Model file for the job. Use its own axes, mm. A direction names the side the tool comes from. Give positions to 0.01 mm unless a question says otherwise; leave off trailing zeros. Order: outer loops, then holes, each group sorted by start corner. A loop starts at its lowest first (then second) coordinate and runs counter-clockwise, first axis right, second up. Notation, with made-up numbers: M 26,7.25 L 76,7.25 A29 cw 76,35.25 Z; hole C 60.25,40 d10. An arc over 180 degrees is marked long. Return JSON: item names as keys, results as strings. Group by question number.
1. Slice it at B-B on z = 3.75. List the corners of the cut face in (x, y), then the cut area to 3 significant figures.
2. Two-plate mould, pull along Y, no slides. Class faces 1 (the face through (0, 42.5, 12)), 2 (the face through (26, -1, 10)), 3 (the face through (0, -1, 18)): released by +Y, released by -Y, zero draft, split by the parting line, or undercut.
3. 3-axis set-ups, long thin cutter, end or side, ignore diameter. For faces 4 (the face through (25, 1, -1)), 5 (the face through (0, 1, 20)), 6 (the face through (-25, 1, -1)), 7 (the face through (-6, -41.5, 15)): which of +Z, -Z, +X, -X, +Y, -Y reach the whole face in a straight line?
4. Pin check, flat tips, straight feed: pin 1 (0.5 mm diameter, centred on x = -3.5, y = 42, fed in from -Z); pin 2 (1.1 mm diameter, centred on x = -24.5, z = -1.5, fed in from -Y); pin 3 (4 mm diameter, centred on x = 3.5, z = 12.5, fed in from -Y). Stop position of each tip, or through.
5. Slice it at C-C on y = -8.5. List the corners of the cut face in (x, z).
6. Slice it at A-A on x = 17. List the corners of the cut face in (y, z), then the cut area to 3 significant figures.
7. Slice it at D-D on z = 11.5. List the corners of the cut face in (x, y).
8. Wall check: probe 1 along Y at (x, z) = (19, 17.75); probe 2 along X at (y, z) = (-7, 16); probe 3 along X at (y, z) = (20, -0.5). Give the ranges that are in metal, low to high. Write a range as [from, to].
from build123d import *

# Parameters (mm, degrees)
F0_W     = 52
F0_H     = 85
F1_DEPTH = 20
F2_W     = 48
F2_H     = 83
F3_DEPTH = 18
F4_W     = 1
F4_H     = 83
F5_DEPTH = 3
F7_DEPTH = 25
F9_DEPTH = 25


with BuildPart() as f1:
    # F0 (on Top) → F1 (new body)
    with BuildSketch(Plane.XY):
        Rectangle(F0_W, F0_H)
    extrude(amount=F1_DEPTH)

    # F2 (on face) → F3 (cut)
    with BuildSketch(Plane(origin=(0, 0, 0), x_dir=(1, 0, 0), z_dir=(0, 0, -1))):
        Rectangle(F2_W, F2_H)
    extrude(amount=-F3_DEPTH, mode=Mode.SUBTRACT)

    # F4 (on face) → F5 (join)
    with BuildSketch(Plane(origin=(0, 0, 0), x_dir=(1, 0, 0), z_dir=(0, 0, -1))):
        with Locations((-24.5, 0)):
            Rectangle(F4_W, F4_H)
        with Locations((24.5, 0)):
            Rectangle(F4_W, F4_H)
    extrude(amount=F5_DEPTH)

    # F6 (on face) → F7 (cut)
    with BuildSketch(Plane(origin=(0, 42.5, 0), x_dir=(-1, 0, 0), z_dir=(0, 1, 0))):
        Polygon((-20, 0), (0, 0), (20, 0), (20, 9), (-20, 9), align=None)
    extrude(amount=-F7_DEPTH, mode=Mode.SUBTRACT)

    # F8 (on face) → F9 (cut)
    with BuildSketch(Plane.XZ.offset(42.5)):
        with BuildLine():
            ThreePointArc((10.5, 5), (7.424621, 12.424621), (0, 15.5))
            ThreePointArc((0, 15.5), (-9.020809, 10.373546), (-9.233093, 0))
            Line((-9.233093, 0), (9.233093, 0))
            ThreePointArc((9.233093, 0), (10.178346, 2.420996), (10.5, 5))
        make_face()
    extrude(amount=-F9_DEPTH, mode=Mode.SUBTRACT)


solid = f1.part
Result:
{
 "1": {"outline": "M -26,-42.5 L -10.43,-42.5 L -10.43,-41.5 L -24,-41.5 L -24,41.5 L -20,41.5 L -20,42.5 L -26,42.5 Z; M 10.43,-42.5 L 26,-42.5 L 26,42.5 L 20,42.5 L 20,41.5 L 24,41.5 L 24,-41.5 L 10.43,-41.5 Z", "area": "375 mm2"},
 "2": {"face 1": "released by +Y", "face 2": "zero draft", "face 3": "undercut"},
 "3": {"face 4": "-Z, +X, +Y, -Y", "face 5": "+Z, +X, -X, +Y, -Y", "face 6": "-Z, -X, +Y, -Y", "face 7": "-Z"},
 "4": {"pin 1": "stops at z = 9", "pin 2": "stops at y = -41.5", "pin 3": "stops at y = 41.5"},
 "5": {"outline": "M -26,0 L -25,0 L -25,-3 L -24,-3 L -24,18 L 24,18 L 24,-3 L 25,-3 L 25,0 L 26,0 L 26,20 L -26,20 Z"},
 "6": {"outline": "M -42.5,0 L -41.5,0 L -41.5,18 L 41.5,18 L 41.5,9 L 42.5,9 L 42.5,20 L -42.5,20 Z", "area": "197 mm2"},
 "7": {"outline": "M -26,-42.5 L -8.25,-42.5 L -8.25,-41.5 L -24,-41.5 L -24,41.5 L 24,41.5 L 24,-41.5 L 8.25,-41.5 L 8.25,-42.5 L 26,-42.5 L 26,42.5 L -26,42.5 Z"},
 "8": {"probe 1": "y = [-42.5, -41.5], [41.5, 42.5]", "probe 2": "x = [-26, -24], [24, 26]", "probe 3": "x = [-25, -24], [24, 25]"}
}
